```python
from build123d import *

# Parameters (mm, degrees)
CYLINDER006_R      = 2.15
CYLINDER006_DEPTH  = 10
CYLINDER005_R      = 2.15
CYLINDER005_DEPTH  = 10
BOX012_W           = 4.3
BOX012_H           = 4
BOX012_DEPTH       = 10
CYLINDER008_R      = 5
CYLINDER008_DEPTH  = 10
BOX013_W           = 10
BOX013_H           = 4
BOX013_DEPTH       = 10
CYLINDER007_R      = 5
CYLINDER007_DEPTH  = 10
BOX010_W           = 1
BOX010_H           = 16
BOX010_DEPTH       = 2
BOX009_W           = 40
BOX009_H           = 30
BOX009_DEPTH       = 5
BOX011_W           = 1
BOX011_H           = 16
BOX011_DEPTH       = 2
CHAMFER003002_SIZE = 1
CHAMFER003003_SIZE = 0.4


with BuildPart() as cylinder006:
    # Cylinder006 → Cylinder006 (new body)
    with BuildSketch(Plane(origin=(0, -8, 0), x_dir=(1, 0, 0), z_dir=(0, 0, 1))):
        Circle(CYLINDER006_R)
    extrude(amount=CYLINDER006_DEPTH)


with BuildPart() as cylinder005:
    # Cylinder005 → Cylinder005 (new body)
    with BuildSketch(Plane(origin=(0, -4, 0), x_dir=(1, 0, 0), z_dir=(0, 0, 1))):
        Circle(CYLINDER005_R)
    extrude(amount=CYLINDER005_DEPTH)


with BuildPart() as fusion009003:
    # Box012 → Box012 (new body)
    with BuildSketch(Plane(origin=(-2.15, -8, 0), x_dir=(1, 0, 0), z_dir=(0, 0, 1))):
        with Locations((2.15, 2)):
            Rectangle(BOX012_W, BOX012_H)
    extrude(amount=BOX012_DEPTH)

    # Fusion009003: union Cylinder006, Cylinder005
    add(cylinder006.part)
    add(cylinder005.part)


with BuildPart() as cylinder008:
    # Cylinder008 → Cylinder008 (new body)
    with BuildSketch(Plane(origin=(0, -8, 0), x_dir=(1, 0, 0), z_dir=(0, 0, 1))):
        Circle(CYLINDER008_R)
    extrude(amount=CYLINDER008_DEPTH)


with BuildPart() as cube013:
    # Box013 → Box013 (new body)
    with BuildSketch(Plane(origin=(-5, -8, 0), x_dir=(1, 0, 0), z_dir=(0, 0, 1))):
        with Locations((5, 2)):
            Rectangle(BOX013_W, BOX013_H)
    extrude(amount=BOX013_DEPTH)


with BuildPart() as fusion009005:
    # Cylinder007 → Cylinder007 (new body)
    with BuildSketch(Plane(origin=(0, -4, 0), x_dir=(1, 0, 0), z_dir=(0, 0, 1))):
        Circle(CYLINDER007_R)
    extrude(amount=CYLINDER007_DEPTH)

    # Fusion009004: union Cylinder008, Cube013
    add(cylinder008.part)
    add(cube013.part)


with BuildPart() as fusion009005_1:
    # Fusion009004 placement: moved
    add(fusion009005.part.moved(Location((0, 0, 10))))

    # Fusion009005: union Fusion009003
    add(fusion009003.part)


with BuildPart() as fusion009005_2:
    # Fusion009005 placement: moved
    add(fusion009005_1.part.moved(Location((0, 0, 17.5))))


with BuildPart() as cube010:
    # Box010 → Box010 (new body)
    with BuildSketch(Plane(origin=(-17.5, -15, 24), x_dir=(1, 0, 0), z_dir=(0, 0, 1))):
        with Locations((0.5, 8)):
            Rectangle(BOX010_W, BOX010_H)
    extrude(amount=BOX010_DEPTH)


with BuildPart() as cube009:
    # Box009 → Box009 (new body)
    with BuildSketch(Plane(origin=(-20, -15, 25), x_dir=(1, 0, 0), z_dir=(0, 0, 1))):
        with Locations((20, 15)):
            Rectangle(BOX009_W, BOX009_H)
    extrude(amount=BOX009_DEPTH)


with BuildPart() as cut006:
    # Box011 → Box011 (new body)
    with BuildSketch(Plane(origin=(16.5, -15, 24), x_dir=(1, 0, 0), z_dir=(0, 0, 1))):
        with Locations((0.5, 8)):
            Rectangle(BOX011_W, BOX011_H)
    extrude(amount=BOX011_DEPTH)

    # Fusion009002: union Cube010, Cube009
    add(cube010.part)
    add(cube009.part)

    # Chamfer003002
    chamfer003002_edges = [cut006.edges().sort_by_distance(p)[0] for p in [
        (20, 0, 30),
        (-20, 0, 30),
    ]]
    chamfer(chamfer003002_edges, length=CHAMFER003002_SIZE)

    # Chamfer003003
    chamfer003003_edges = [cut006.edges().sort_by_distance(p)[0] for p in [
        (20, 0, 25),
        (-20, 0, 25),
    ]]
    chamfer(chamfer003003_edges, length=CHAMFER003003_SIZE)

    # Cut006: cut Fusion009005
    add(fusion009005_2.part, mode=Mode.SUBTRACT)


solid = cut006.part
```
Could you check a few things on this model? Use its own coordinates, in mm. A direction names the side the tool comes from. Coordinates: 2 decimals unless noted, no trailing zeros. Order: outer loops, then holes, each group sorted by start corner. A loop starts at its lowest first (then second) coordinate and runs counter-clockwise, first axis right, second up. Notation, with made-up numbers: M -0.5,6.25 L 7.5,6.25 A20 ccw 7.5,12.25 Z; hole C 56.5,77 d5. An arc over 180 degrees is marked long. Use a Markdown table: item, result. Add a question column.
Q1. I want a section at B-B on y = -3. List the corners of the cut face in (x, z) for me.
Q2. Which directions (+Z, -Z, +X, -X, +Y, -Y) give clear straight access to the entire face, cutting with the end or side of a thin tool? Please do faces 1 (the flat face through (17.5, -7.1, 24.5)), 2 (the flat face through (16.5, -7.1, 24.5)), 3 (the flat face through (-17.5, -7.1, 24.5)), 4 (the flat face through (5, -6, 29)).
Q3. If I drill on L1, parallel to Y at x = 0, z = 29.2; L2, parallel to Z at x = 15, y = -4; L3, parallel to X at y = -0.75, z = 24.3, over which ranges is the centre line in solid material (lowest first)?
Q4. I want a section at D-D on y = -12.5. List the corners of the cut face in (x, z) for me.
Q5. I want a section at A-A on z = 25.95. List the corners of the cut face in (x, y) for me, then the cut area to 3 significant figures.
Q6. I want a section at C-C on x = 3. List the corners of the cut face in (y, z) for me.
Q7. We'd pull the mould along X, two halves only. Please class faces 5 (the flat face through (-17, -7, 24)), 6 (the flat face through (-20, 0, 27)), 7 (the cylindrical face through (-0.05, -10.15, 26.23)): pulls with the +X half, pulls with the -X half, needs draft (parallel to the pull), parting line crosses it, or undercut.
Q8. I'm going to push flat-ended pins straight in: pin 1 (9 mm diameter, centred on x = -8.5, y = -5.5, fed in from -Z); pin 2 (8 mm diameter, centred on x = 0, y = -7.5, fed in from +Z); pin 3 (1.1 mm diameter, centred on y = -6.5, z = 24.5, fed in from +X). Where does each tip first touch, or does it pass through?
Checked values:
| question | item | result |
|---|---|---|
| 1 | outline | M -20,25.4 L -19.6,25 L -17.5,25 L -17.5,24 L -16.5,24 L -16.5,25 L -1.9,25 L -1.9,27.5 L -4.9,27.5 L -4.9,30 L -19,30 L -20,29 Z; M 1.9,25 L 16.5,25 L 16.5,24 L 17.5,24 L 17.5,25 L 19.6,25 L 20,25.4 L 20,29 L 19,30 L 4.9,30 L 4.9,27.5 L 1.9,27.5 Z |
| 2 | face 1 | -Z, +X, +Y, -Y |
| 2 | face 2 | -Z, +Y, -Y |
| 2 | face 3 | -Z, -X, +Y, -Y |
| 2 | face 4 | +Z |
| 3 | L1 | -15 to -13, 1 to 15 |
| 3 | L2 | 25 to 30 |
| 3 | L3 | -17.5 to -16.5, 16.5 to 17.5 |
| 4 | outline | M -20,25.4 L -19.6,25 L -17.5,25 L -17.5,24 L -16.5,24 L -16.5,25 L 16.5,25 L 16.5,24 L 17.5,24 L 17.5,25 L 19.6,25 L 20,25.4 L 20,29 L 19,30 L 2.18,30 L 2.18,27.5 L -2.18,27.5 L -2.18,30 L -19,30 L -20,29 Z |
| 5 | outline | M -20,-15 L 20,-15 L 20,15 L -20,15 Z; hole M -2.15,-8 A2.15 ccw 2.15,-8 L 2.15,-4 A2.15 ccw -2.15,-4 Z |
| 5 | area | 1,170 mm² |
| 6 | outline | M -15,25 L 15,25 L 15,30 L 0,30 L 0,27.5 L -12,27.5 L -12,30 L -15,30 Z |
| 7 | face 5 | needs draft |
| 7 | face 6 | pulls with the -X half |
| 7 | face 7 | undercut |
| 8 | pin 1 | z = 25 |
| 8 | pin 2 | z = 27.5 |
| 8 | pin 3 | x = 19.65 |
